Here's how the part is built. I have some questions about the finished solid (model axes, mm). Coordinates: 2 decimals unless noted, no trailing zeros. Write each loop counter-clockwise with the first axis right and the second up, starting at its lowest first coordinate (ties: lowest second). Pieces come first, ordered by that corner, then holes. Notation, with made-up numbers: (-25, 22.25) - (30, 22.25) arc R14 cw to (30, 30.25) - close; hole circle Ø8 at (70, 56). An arc over 180 degrees is marked (long way). Answer in a Markdown table with one row per item. Add a question column.
Item 1: If I drill on probe 1 along X at (y, z) = (-17.25, 383.5); probe 2 along Z at (x, y) = (80.5, -1.5); probe 3 along Z at (x, y) = (270, -21.5), over which ranges is the centre line in solid material (lowest first)? Write a range as from..to.
Item 2: I'm going to push flat-ended pins straight in: pin 1 (1 mm diameter, centred on x = 292, y = -16, fed in from +Z); pin 2 (1 mm diameter, centred on y = -5.5, z = 280.5, fed in from -X); pin 3 (4 mm diameter, centred on y = -15.5, z = 275.5, fed in from +X). Where does each tip first touch, or does it pass through?
Item 3: Imagine slicing it at C-C (z = 173.5). Please give me the cut outline in (x, y).
Item 4: Imagine slicing it at D-D (x = 98.5). Please give me the cut outline in (y, z).
Item 5: Imagine slicing it at B-B (x = 264). Please give me the cut outline in (y, z), plus the area to 3 significant figures.
from build123d import *

# Parameters (mm, degrees)
F1_DEPTH = 25


with BuildPart() as f1:
    # F0 (on Front) → F1 (new body)
    with BuildSketch(Plane.XZ):
        with BuildLine():
            ThreePointArc((141.238138, 444.997787), (112.749463, 429.773668), (81.014585, 423.750718))
            ThreePointArc((81.014585, 423.750718), (65.741999, 411.97311), (49.000544, 402.397745))
            ThreePointArc((49.000544, 402.397745), (33.218565, 392.066346), (20.588335, 378.056139))
            ThreePointArc((20.588335, 378.056139), (9.877069, 357.822031), (4.194495, 335.644143))
            ThreePointArc((4.194495, 335.644143), (6.529558, 291.46217), (24.733176, 251.136899))
            ThreePointArc((24.733176, 251.136899), (39.945084, 220.899663), (45.972874, 187.592631))
            ThreePointArc((45.972874, 187.592631), (45.912459, 175.6279), (44.882946, 163.70739))
            ThreePointArc((44.882946, 163.70739), (87.378349, 115.792993), (44.882946, 67.878596))
            ThreePointArc((44.882946, 67.878596), (46.748425, 57.916658), (44.882946, 47.95472))
            ThreePointArc((44.882946, 47.95472), (41.39103, 40.901455), (36.6995, 34.582313))
            ThreePointArc((36.6995, 34.582313), (32.469146, 28.993084), (29.186027, 22.799822))
            ThreePointArc((29.186027, 22.799822), (25.823713, 11.635955), (25.087768, 0))
            Line((25.087768, 0), (308.352295, 0))
            ThreePointArc((308.352295, 0), (307.61635, 11.635955), (304.254036, 22.799822))
            ThreePointArc((304.254036, 22.799822), (300.970917, 28.993084), (296.740563, 34.582313))
            ThreePointArc((296.740563, 34.582313), (292.049033, 40.901455), (288.557117, 47.95472))
            ThreePointArc((288.557117, 47.95472), (286.691638, 57.916658), (288.557117, 67.878596))
            ThreePointArc((288.557117, 67.878596), (246.061714, 115.792993), (288.557117, 163.70739))
            ThreePointArc((288.557117, 163.70739), (287.527604, 175.6279), (287.467189, 187.592631))
            ThreePointArc((287.467189, 187.592631), (293.494979, 220.899663), (308.706887, 251.136899))
            ThreePointArc((308.706887, 251.136899), (326.910505, 291.46217), (329.245568, 335.644143))
            ThreePointArc((329.245568, 335.644143), (323.562994, 357.822031), (312.851728, 378.056139))
            ThreePointArc((312.851728, 378.056139), (300.221498, 392.066346), (284.439519, 402.397745))
            ThreePointArc((284.439519, 402.397745), (267.698064, 411.97311), (252.425478, 423.750718))
            ThreePointArc((252.425478, 423.750718), (220.6906, 429.773668), (192.201925, 444.997787))
            ThreePointArc((192.201925, 444.997787), (166.720032, 453.476058), (141.238138, 444.997787))
        make_face()
        with BuildLine():
            ThreePointArc((166.720032, 300.744148), (177.104622, 308.249052), (189.916627, 308.123254))
            ThreePointArc((189.916627, 308.123254), (200.288352, 300.033358), (203.399401, 287.252887))
            ThreePointArc((203.399401, 287.252887), (198.645247, 272.102034), (188.17311, 260.16534))
            ThreePointArc((188.17311, 260.16534), (177.878406, 253.598127), (166.720032, 248.638297))
            ThreePointArc((166.720032, 248.638297), (155.561657, 253.598127), (145.266953, 260.16534))
            ThreePointArc((145.266953, 260.16534), (134.794816, 272.102034), (130.040662, 287.252887))
            ThreePointArc((130.040662, 287.252887), (133.151711, 300.033358), (143.523436, 308.123254))
            ThreePointArc((143.523436, 308.123254), (156.335441, 308.249052), (166.720032, 300.744148))
        make_face(mode=Mode.SUBTRACT)
    extrude(amount=F1_DEPTH)


solid = f1.part
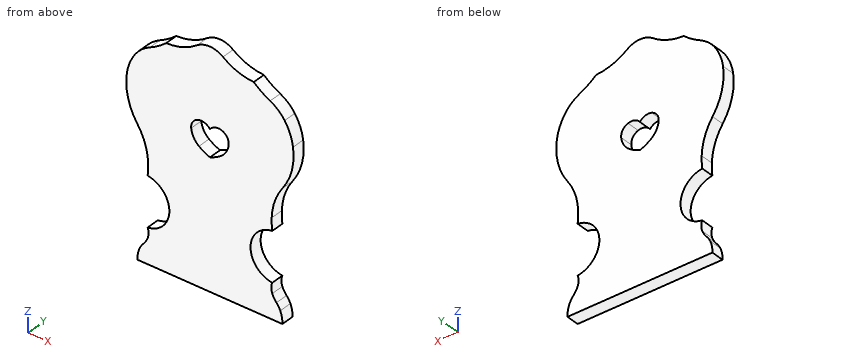
Here are the results:
| question | item | result |
|---|---|---|
| 1 | probe 1 | x = 24.74..308.7 |
| 1 | probe 2 | z = 0..90.96, 140.62..423.3 |
| 1 | probe 3 | z = 0..74.11, 157.48..410.47 |
| 2 | pin 1 | stops at z = 398.49 |
| 2 | pin 2 | stops at x = 9.58 |
| 2 | pin 3 | stops at x = 322.6 |
| 3 | outline | (45.8, -25) - (287.64, -25) - (287.64, 0) - (45.8, 0) - close |
| 4 | outline | (-25, 0) - (0, 0) - (0, 425.83) - (-25, 425.83) - close |
| 5 | outline | (-25, 0) - (0, 0) - (0, 78.25) - (-25, 78.25) - close; (-25, 153.34) - (0, 153.34) - (0, 414.53) - (-25, 414.53) - close |
| 5 | area | 8,490 mm2 |
